For this review, take the finished solid that the model builds, in its own axes (mm). Face numbers are marked on the shaded views. A direction names the side the tool comes from. Give positions to 0.01 mm unless a question says otherwise; leave off trailing zeros. Order: outer loops, then holes, each group sorted by start corner. A loop starts at its lowest first (then second) coordinate and runs counter-clockwise, first axis right, second up.
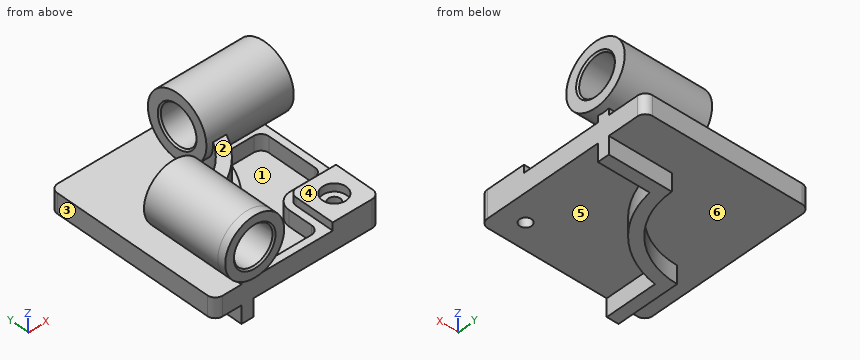
from build123d import *

# Parameters (mm, degrees)
F0_W            = 210
F0_H            = 225
F1_DEPTH        = 12.5
F3_DEPTH        = 47.5
F4_R            = 37.5
F5_DEPTH        = 10
F5_DEPTH_BACK   = 101
F6_R            = 40
F7_DEPTH        = 10
F7_DEPTH_BACK   = 101
F8_W            = 60
F8_H            = 60
F9_DEPTH        = 10
F10_R           = 10
F12_DEPTH       = 20
F14_D           = 1.5
F14_CBORE_D     = 3
F14_CBORE_DEPTH = 1
F16_D           = 15
F16_CBORE_D     = 30
F16_CBORE_DEPTH = 10
F17_R           = 10
F18_R           = 24.5
F19_DEPTH       = 235.001
F20_R           = 24.5
F21_DEPTH       = 220.001
F22_SIZE        = 2


with BuildPart() as f1:
    # F0 (on Top) → F1 (new body, symmetric)
    with BuildSketch(Plane.XY):
        Rectangle(F0_W, F0_H)
    extrude(amount=F1_DEPTH, both=True)

    # F2 (on face) → F3 (join, symmetric)
    with BuildSketch(Plane.XY.offset(12.5)):
        with BuildLine():
            Line((105, 48.5), (105, 63.5))
            Line((105, 63.5), (25, 63.5))
            ThreePointArc((25, 63.5), (-3.1177490061, -4.3822509939), (-71, -32.5))
            Line((-71, -32.5), (-71, -112.5))
            Line((-71, -112.5), (-56, -112.5))
            Line((-56, -112.5), (-56, -46.4818166789))
            ThreePointArc((-56, -46.4818166789), (7.4888527117, -14.9888527117), (38.9818166789, 48.5))
            Line((38.9818166789, 48.5), (105, 48.5))
        make_face()
    extrude(amount=F3_DEPTH, both=True)

    # F4 (on face) → F5 (join, two sides)
    with BuildSketch(Plane.XZ.offset(112.5)) as f5_sk:
        with Locations((-63.5, 60)):
            Circle(F4_R)
    extrude(amount=F5_DEPTH)
    extrude(f5_sk.sketch, amount=-F5_DEPTH_BACK)

    # F6 (on face) → F7 (join, two sides)
    with BuildSketch(Plane.YZ.offset(105)) as f7_sk:
        with Locations((56, 60)):
            Circle(F6_R)
    extrude(amount=F7_DEPTH)
    extrude(f7_sk.sketch, amount=-F7_DEPTH_BACK)

    # F8 (on face) → F9 (join)
    with BuildSketch(Plane.XY.offset(12.5)):
        with Locations((75, -82.5)):
            Rectangle(F8_W, F8_H)
    extrude(amount=F9_DEPTH)

    # F10
    f10_edges = [f1.edges().sort_by_distance(p)[0] for p in [
        (45, -52.5, 17.5),
    ]]
    fillet(f10_edges, radius=F10_R)

    # F11 (on face) → F12 (cut)
    with BuildSketch(Plane.XY.offset(12.5)):
        with BuildLine():
            ThreePointArc((46.5755076536, 39.5), (13.8528137424, -21.3528137424), (-47, -54.0755076536))
            Line((-47, -54.0755076536), (-47, -103.5))
            Line((-47, -103.5), (36, -103.5))
            Line((36, -103.5), (36, -62.5))
            ThreePointArc((36, -62.5), (41.5649711575, -49.0649711575), (55, -43.5))
            Line((55, -43.5), (96, -43.5))
            Line((96, -43.5), (96, 39.5))
            Line((96, 39.5), (46.5755076536, 39.5))
        make_face()
    extrude(amount=-F12_DEPTH, mode=Mode.SUBTRACT)

    # F14 (through all)
    with Locations(Plane.XY.offset(22.5)):
        with Locations((75, -82.5)):
            CounterBoreHole(F14_D / 2, F14_CBORE_D / 2, F14_CBORE_DEPTH)

    # F16 (through all)
    with Locations(Plane.XY.offset(22.5)):
        with Locations((75, -82.5)):
            CounterBoreHole(F16_D / 2, F16_CBORE_D / 2, F16_CBORE_DEPTH)

    # F17
    f17_edges = [f1.edges().sort_by_distance(p)[0] for p in [
        (-47, -54.075508, 2.5),
        (46.575508, 39.5, 2.5),
        (-105, -112.5, 0),
        (105, -112.5, 5),
        (105, 112.5, 0),
        (36, -103.5, 2.5),
        (96, -43.5, 2.5),
        (-47, -103.5, 2.5),
        (96, 39.5, 2.5),
        (-105, 112.5, 0),
    ]]
    fillet(f17_edges, radius=F17_R)

    # F18 (on face) → F19 (cut, through all)
    with BuildSketch(Plane.XZ.offset(122.5)):
        with Locations((-63.5, 60)):
            Circle(F18_R)
    extrude(amount=-F19_DEPTH, mode=Mode.SUBTRACT)

    # F20 (on face) → F21 (cut, through all)
    with BuildSketch(Plane.YZ.offset(115)):
        with Locations((56, 60)):
            Circle(F20_R)
    extrude(amount=-F21_DEPTH, mode=Mode.SUBTRACT)

    # F22
    f22_edges = [f1.edges().sort_by_distance(p)[0] for p in [
        (-88, -122.5, 60),
        (115, 31.5, 60),
        (4, 31.5, 60),
        (-88, -11.5, 60),
    ]]
    chamfer(f22_edges, length=F22_SIZE)


solid = f1.part
1) We need section C-C on z = -23.5. Give the boundary of the cut face in (x, y).
Answer sheet:
outline: (-71, -112.5) - (-56, -112.5) - (-56, -46.48) arc R111 ccw to (38.98, 48.5) - (105, 48.5) - (105, 63.5) - (25, 63.5) arc R96 cw to (-71, -32.5) - close
2) We need section A-A on y = -82.5. Give the boundary of the cut face in (x, z), then the cut area to 3 significant figures.
Answer sheet:
outline: (-105, -12.5) - (-71, -12.5) - (-71, -35) - (-56, -35) - (-56, -12.5) - (67.5, -12.5) - (67.5, 12.5) - (60, 12.5) - (60, 22.5) - (45, 22.5) - (45, 12.5) - (36, 12.5) - (36, -7.5) - (-47, -7.5) - (-47, 12.5) - (-56, 12.5) - (-56, 23.26) arc R37.5 ccw (long way) to (-71, 23.26) - (-71, 12.5) - (-105, 12.5) - close; (82.5, -12.5) - (105, -12.5) - (105, 22.5) - (90, 22.5) - (90, 12.5) - (82.5, 12.5) - close; hole circle Ø49 at (-63.5, 60)
area: 6,540 mm2
3) We need section B-B on x = 75. Give the boundary of the cut face in (y, z), then the cut area to 3 significant figures.
Answer sheet:
outline: (-112.5, -12.5) - (-90, -12.5) - (-90, 12.5) - (-97.5, 12.5) - (-97.5, 22.5) - (-112.5, 22.5) - close; (-75, -12.5) - (48.5, -12.5) - (48.5, -35) - (63.5, -35) - (63.5, -12.5) - (112.5, -12.5) - (112.5, 12.5) - (63.5, 12.5) - (63.5, 20.71) arc R40 ccw (long way) to (48.5, 20.71) - (48.5, 12.5) - (39.5, 12.5) - (39.5, -7.5) - (-43.5, -7.5) - (-43.5, 12.5) - (-52.5, 12.5) - (-52.5, 22.5) - (-67.5, 22.5) - (-67.5, 12.5) - (-75, 12.5) - close; hole circle Ø49 at (56, 60)
area: 7,480 mm2
4) Clearance check with flat-ended pins moving along their axes: pin 1 (18 mm diameter, centred on x = 75, y = -82.5, fed in from -Z); pin 2 (12 mm diameter, centred on x = 75, y = -82.5, fed in from -Z); pin 3 (4 mm diameter, centred on x = -77.5, y = -21.5, fed in from +Z); pin 4 (1 mm diameter, centred on y = -94, z = 20, fed in from -X). State where each tip first meets the part, or that it passes through.
Answer sheet:
pin 1: stops at z = -12.5
pin 2: passes through
pin 3: stops at z = 95.53
pin 4: stops at x = -71
5) To check wall thickness, follow line 1 (Z direction, x = 20, y = 56); line 2 (X direction, y = -82, z = -5); line 3 (Y direction, x = 75, z = -3.5). State the ranges of each line that lie inside material, in increasing order.
Answer sheet:
line 1: z = -12.5 to 12.5, 20 to 35.5, 84.5 to 100
line 2: x = -105 to -47, 36 to 67.52, 82.48 to 105
line 3: y = -112.5 to -90, -75 to -43.5, 39.5 to 112.5
6) Tool access review of the marked faces 4, 5 and 6: name each direction out of +Z, -Z, +X, -X, +Y, -Y from which nothing blocks a thin tool from reaching the whole face with its end or side.
Answer sheet:
face 4: +Z, +X, -Y
face 5: -Z, +X, -Y
face 6: -Z, -X, +Y
7) We need section D-D on x = 20.5. Give the boundary of the cut face in (y, z).
Answer sheet:
outline: (-112.5, -12.5) - (0.66, -12.5) - (0.66, -35) - (34.45, -35) - (34.45, -12.5) - (112.5, -12.5) - (112.5, 12.5) - (34.45, 12.5) - (34.45, 26.3) arc R40 ccw (long way) to (16, 60) - (0.66, 60) - (0.66, 12.5) - (-14.14, 12.5) - (-14.14, -7.5) - (-103.5, -7.5) - (-103.5, 12.5) - (-112.5, 12.5) - close; hole circle Ø49 at (56, 60)
8) Draft analysis for pull direction Z (two halves, no side actions). For the marked faces 1, 2 and 3, state which applies: +Z half, -Z half, draft (parallel to the pull), parting line (faces both ways), or undercut.
Answer sheet:
face 1: undercut
face 2: +Z half
face 3: draft
